Here's how the part is built. I have some questions about the finished solid (model axes, mm). Coordinates: 2 decimals unless noted, no trailing zeros. Loops run counter-clockwise (first coordinate to the right, second up) from the corner with the lowest first, then second, coordinate; pieces in that order, holes last. Notation, with made-up numbers: M 43,51.5 L 91,51.5 A17 ccw 91,84.5 Z; hole C 25.5,26 d10. An arc over 180 degrees is marked long. Use one line per item in the form item = value. Start each with the question number.
(1) Imagine slicing it at A-A, the plane z = 72. Please give me the cut outline in (x, y), and give its area (3 significant figures).
(2) Please list where these lines run through material, in increasing order: L1, parallel to Y at x = -8.5, z = 140.5; L2, parallel to Y at x = 7.5, z = 234; L3, parallel to X at y = -8.5, z = 13.
(3) Imagine slicing it at D-D, the plane y = -5.5. Please give me the cut outline in (x, z).
(4) Imagine slicing it at C-C, the plane z = 264. Please give me the cut outline in (x, y).
(5) Imagine slicing it at B-B, the plane x = -3. Please give me the cut outline in (y, z), and give its area (3 significant figures).
(6) Will this pin go through, and if not, where does the flat tip stop? P1, Ø3, axis at x = 7.5, y = -9.5, coming from the -Z side.
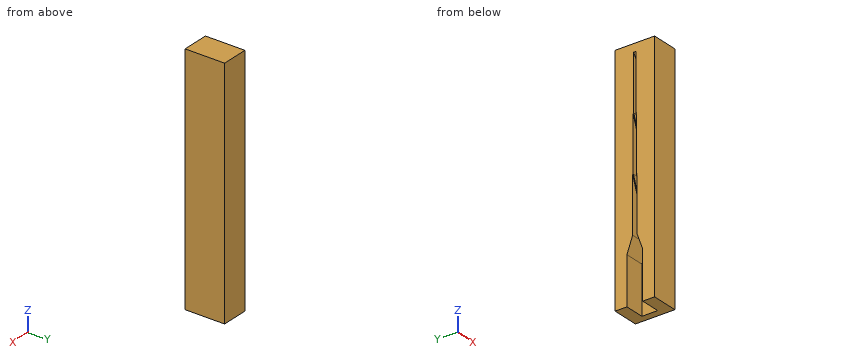
```python
from build123d import *

# Parameters (mm, degrees)
SKETCH1_W           = 34
SKETCH1_H           = 50
BOSS_EXTRUDE1_DEPTH = 300
SKETCH3_W           = 70
SKETCH3_H           = 3
CUT_EXTRUDE1_DEPTH  = 25
SKETCH4_W           = 70
SKETCH4_H           = 4.5
CUT_EXTRUDE2_DEPTH  = 25
SKETCH5_W           = 70
SKETCH5_H           = 5.5
CUT_EXTRUDE3_DEPTH  = 25
SKETCH6_W           = 60
SKETCH6_H           = 20
CUT_EXTRUDE4_DEPTH  = 25
BOSS_EXTRUDE2_DEPTH = 1
BOSS_EXTRUDE3_DEPTH = 1
BOSS_EXTRUDE4_DEPTH = 3


with BuildPart() as part:
    # Sketch1 → Boss-Extrude1 (new body)
    with BuildSketch(Plane.XY):
        Rectangle(SKETCH1_W, SKETCH1_H)
    extrude(amount=BOSS_EXTRUDE1_DEPTH)

    # Sketch3 → Cut-Extrude1 (cut)
    with BuildSketch(Plane.ZY.offset(17)):
        with Locations((255, 0)):
            Rectangle(SKETCH3_W, SKETCH3_H)
    extrude(amount=-CUT_EXTRUDE1_DEPTH, mode=Mode.SUBTRACT)

    # Sketch4 → Cut-Extrude2 (cut)
    with BuildSketch(Plane.ZY.offset(17)):
        with Locations((185, 0)):
            Rectangle(SKETCH4_W, SKETCH4_H)
    extrude(amount=-CUT_EXTRUDE2_DEPTH, mode=Mode.SUBTRACT)

    # Sketch5 → Cut-Extrude3 (cut)
    with BuildSketch(Plane.ZY.offset(17)):
        with Locations((115, 0)):
            Rectangle(SKETCH5_W, SKETCH5_H)
    extrude(amount=-CUT_EXTRUDE3_DEPTH, mode=Mode.SUBTRACT)

    # Sketch6 → Cut-Extrude4 (cut)
    with BuildSketch(Plane.ZY.offset(17)):
        with Locations((30, 0)):
            Rectangle(SKETCH6_W, SKETCH6_H)
        Polygon((60, 10), (80, 2.75), (80, -2.75), (60, -10), align=None)
    extrude(amount=-CUT_EXTRUDE4_DEPTH, mode=Mode.SUBTRACT)

    # Sketch7 → Boss-Extrude2 (add)
    with BuildSketch(Plane(origin=(0, 2.75, 0), x_dir=(-1, 0, 0), z_dir=(0, -1, 0))):
        Polygon((-8, -80), (17, -150), (-8, -150), align=None)
    boss_extrude2 = extrude(amount=BOSS_EXTRUDE2_DEPTH)

    # Sketch9 → Boss-Extrude3 (add)
    with BuildSketch(Plane.XZ.offset(-2.25)):
        Polygon((-17, 220), (8, 220), (8, 150), align=None)
    boss_extrude3 = extrude(amount=BOSS_EXTRUDE3_DEPTH)

    # Sketch10 → Boss-Extrude4 (add)
    with BuildSketch(Plane(origin=(0, 1.5, 0), x_dir=(-1, 0, 0), z_dir=(0, -1, 0))):
        Polygon((17, -290), (-8, -250), (-8, -290), align=None)
    extrude(amount=BOSS_EXTRUDE4_DEPTH)

    # Mirror3: Boss-Extrude2, Boss-Extrude3 across plane
    add(boss_extrude2.mirror(Plane.ZX))
    add(boss_extrude3.mirror(Plane.ZX))


solid = part.part
```
Answer:
q1.outline = M -17,-25 L 17,-25 L 17,25 L -17,25 L -17,5.65 L 8,5.65 L 8,-5.65 L -17,-5.65 Z
q1.area = 1,420 mm²
q2.L1 = -25 to -1.75, 1.75 to 25
q2.L2 = -25 to -1.5, 1.5 to 25
q2.L3 = 8 to 17
q3.outline = M -17,72.41 L 8,72.41 L 8,0 L 17,0 L 17,300 L -17,300 Z
q4.outline = M -17,-25 L 17,-25 L 17,25 L -17,25 L -17,1.5 L -0.75,1.5 L -0.75,-1.5 L -17,-1.5 Z
q5.outline = M -25,0 L -10,0 L -10,60 L -2.75,80 L -2.75,110.8 L -1.75,110.8 L -1.75,150 L -2.25,150 L -2.25,180.8 L -1.25,180.8 L -1.25,220 L -1.5,220 L -1.5,267.6 L 1.5,267.6 L 1.5,220 L 1.25,220 L 1.25,180.8 L 2.25,180.8 L 2.25,150 L 1.75,150 L 1.75,110.8 L 2.75,110.8 L 2.75,80 L 10,60 L 10,0 L 25,0 L 25,300 L -25,300 Z
q5.area = 12,900 mm²
q6.P1 = 0
